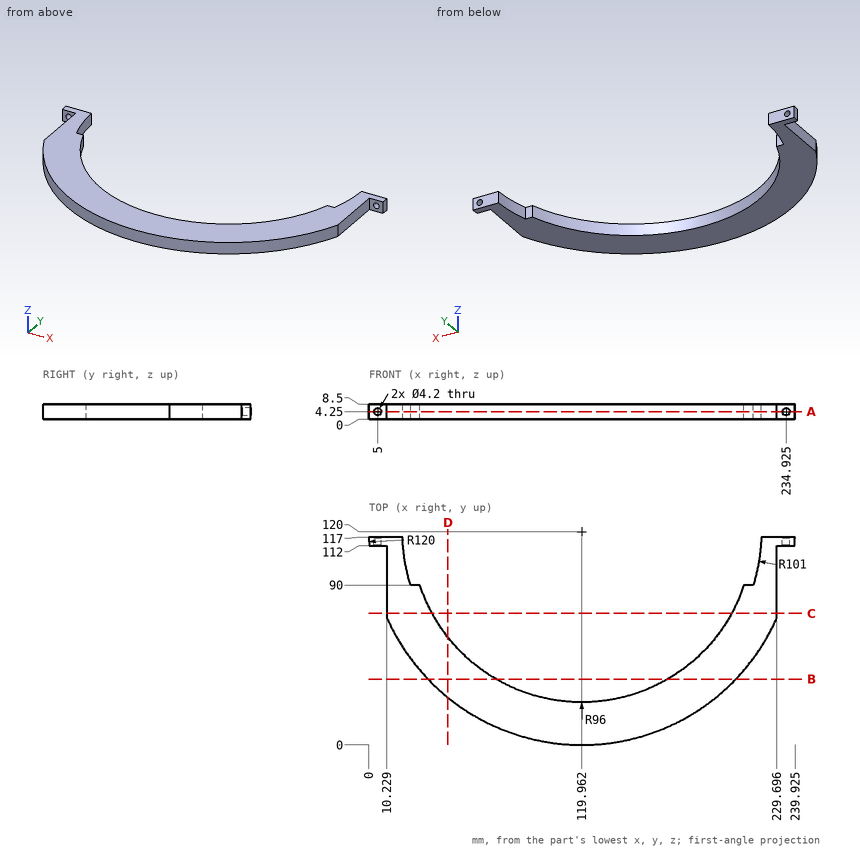
Source: three-view drawing plus pictorial views. Frame: mm from the lowest corner of the part. Coordinates: 2 decimals unless noted, no trailing zeros. Loops run counter-clockwise (first coordinate to the right, second up) from the corner with the lowest first, then second, coordinate; pieces in that order, holes last. Notation, with made-up numbers: (-8, -17.5) -> (-1, -17.5) arc R22 ccw to (-1, -2.5) -> close; hole circle Ø7 at (-25.5, 33.5). An arc over 180 degrees is marked (long way). Answer in a Markdown table with one row per item. Add a question column.
Q1. Contact query for flat-ended pins moving along their axis: pin 1 Ø2 at (y, z) = (89.5, 7.5) entering from -X; pin 2 Ø4 at (x, z) = (26, 2.5) entering from +Y; pin 3 Ø5 at (y, z) = (87, 3.5) entering from +X; pin 4 Ø4 at (x, z) = (5, 4.25) entering from -Y. Output: stop coordinate, or through.
Q2. Section D-D on x = 44.5. Return the cut outline in (y, z).
Q3. Section C-C on y = 74. Return the cut outline in (x, z) (1 decimal).
Q4. Section B-B on y = 37. Return the cut outline in (x, z), and give its area (3 significant figures).
Q5. Section A-A on z = 4.25. Return the cut outline in (x, y) (1 decimal).
Q6. Ray query, line 1 along X through (y, z) = (115.45, 4.25) (1 decimal); line 2 along X through (y, z) = (113.75, 4.25) (1 decimal); line 3 along Y through (x, z) = (117.5, 4.5) (1 decimal). Return the intervals inside material, ascending.
Computed values:
| question | item | result |
|---|---|---|
| 1 | pin 1 | stops at x = 10.23 |
| 1 | pin 2 | stops at y = 90 |
| 1 | pin 3 | stops at x = 229.7 |
| 1 | pin 4 | passes through |
| 2 | outline | (26.7, 0) -> (60.66, 0) -> (60.66, 8.5) -> (26.7, 8.5) -> close |
| 3 | outline | (10.2, 0) -> (35.7, 0) -> (35.7, 8.5) -> (10.2, 8.5) -> close; (204.2, 0) -> (229.7, 0) -> (229.7, 8.5) -> (204.2, 8.5) -> close |
| 4 | outline | (33.3, 0) -> (71.72, 0) -> (71.72, 8.5) -> (33.3, 8.5) -> close; (168.2, 0) -> (206.63, 0) -> (206.63, 8.5) -> (168.2, 8.5) -> close |
| 4 | area | 653 mm^2 |
| 5 | outline | (0, 117) arc R120 ccw to (0.2, 112) -> (2.9, 112) -> (2.9, 117) -> close; (7.1, 112) -> (10.2, 112) -> (10.2, 71.4) arc R120 ccw to (229.7, 71.4) -> (229.7, 112) -> (232.8, 112) -> (232.8, 117) -> (220.9, 117) arc R101 cw to (216.4, 90) -> (211.2, 90) arc R96 cw to (28.8, 90) -> (23.5, 90) arc R101 cw to (19, 117) -> (7.1, 117) -> close; (237, 112) -> (239.7, 112) arc R120 ccw to (239.9, 117) -> (237, 117) -> close |
| 6 | line 1 | x = 0 to 2.9, 7.1 to 19.1, 220.9 to 232.8, 237 to 239.9 |
| 6 | line 2 | x = 0.1 to 2.9, 7.1 to 19.2, 220.8 to 232.8, 237 to 239.8 |
| 6 | line 3 | y = 0 to 24 |
